Geometry check sheet. Reference: the model listing, model coordinates, mm. Give positions to 0.01 mm unless a question says otherwise; leave off trailing zeros. Order: outer loops, then holes, each group sorted by start corner. A loop starts at its lowest first (then second) coordinate and runs counter-clockwise, first axis right, second up.
Autodesk Inventor part; units mm, degrees
ref_plane "YZ Plane" through (0, 0, 0) normal (1, 0, 0) x (0, 1, 0)
ref_plane "XZ Plane" through (0, 0, 0) normal (0, 1, 0) x (-1, 0, 0)
ref_plane "XY Plane" through (0, 0, 0) normal (0, 0, 1) x (1, 0, 0)
sketch "Sketch1" plane through (0, 0, 0) normal (0, 1, 0) x (-1, 0, 0)
  circle A0 centre (0, 0) radius 2.5
  line L0 (-22.4, 0) -> (15.4, 0)
  line L1 (2.5, 0) -> (1.5, 0)
  line L2 (1.5, 0) -> (1.5, -17)
  line L3 (1.5, -17) -> (2.5, -17)
  line L4 (2.5, -17) -> (2.5, 0)
  line L5 (0, 0) -> (-7.0711, -7.0711) construction
  line L6 (0, 0) -> (10, 0) construction
  line L7 (0, 1.5) -> (-17, 1.5)
  line L8 (-17, 1.5) -> (-17, 2.5)
  line L9 (-17, 2.5) -> (0, 2.5)
  line L10 (0, 1.5) -> (0, 2.5)
  dimension "d0" = 5
  dimension "d1" = 1
  dimension "d2" = 17
  dimension "d3" = 10
  dimension "d4" = 135
extrude "Extrusion1" add sketch "Sketch1" along normal blind 60
sketch "Sketch2" plane through (17, 0, 1.5) normal (0, 0, -1) x (-1, 0, 0)
  line L0 (0, 60) -> (15, 60)
  line L1 (7, 60) -> (7, 0) construction
  line L2 (15, 0) -> (0, 0)
  line L3 (0, 0) -> (0, 60)
  point P0 (17, 0)
  point P1 (7, 30)
  point P2 (7, 53)
  point P3 (7, 7)
  dimension "d7" = 7
  dimension "d8" = 30
  dimension "d9" = 7
  dimension "d10" = 7
hole "Hole1" at (10, 30, 1.5) at (10, 53, 1.5) at (10, 7, 1.5) direction (0, 0, 1) diameter 3.4 end through all
sketch "Sketch3" plane through (-1.5, 0, -2) normal (1, 0, 0) x (0, 0, -1)
  line L0 (0, 60) -> (15, 60)
  line L1 (8, 60) -> (8, 0) construction
  line L2 (15, 0) -> (15, 60)
  line L3 (15, 0) -> (0, 0)
  point P0 (-2, 0)
  point P1 (8, 30)
  point P2 (8, 7)
  point P3 (8, 53)
  dimension "d18" = 7
  dimension "d19" = 30
  dimension "d20" = 7
  dimension "d21" = 7
hole "Hole2" at (-1.5, 30, -10) at (-1.5, 7, -10) at (-1.5, 53, -10) direction (-1, 0, 0) diameter 3.4 end through all
properties part number "scharnier"
Item 1: Sectioned sample at C-C (x = 10). Enter the section's corners in (y, z), and give its area (3 significant figures).
Reported:
outline: (0, 1.5) - (5.3, 1.5) - (5.3, 2.5) - (0, 2.5) - close; (8.7, 1.5) - (28.3, 1.5) - (28.3, 2.5) - (8.7, 2.5) - close; (31.7, 1.5) - (51.3, 1.5) - (51.3, 2.5) - (31.7, 2.5) - close; (54.7, 1.5) - (60, 1.5) - (60, 2.5) - (54.7, 2.5) - close
area: 49.8 mm2
Item 2: Draft check along Z on faces 1 (the cylindrical face through (1.732, 29.58, -1.803)), 2 (the cylindrical face through (11.66, 6.63, 2.01)), 3 (the flat face through (-2, 30, -17)). Enter one of: released by +Z, released by -Z, zero draft, split by the parting line, or undercut.
Reported:
face 1: undercut
face 2: zero draft
face 3: released by -Z
Item 3: Gauge pin test, flat ends, axial feed: pin 1 (4.5 mm diameter, centred on x = 12.5, y = 24, fed in from -Z); pin 2 (4 mm diameter, centred on y = 53, z = -10, fed in from +X); pin 3 (5 mm diameter, centred on x = 2, y = 38, fed in from -Z). Record the tip position at first contact, or that the pin passes through.
Reported:
pin 1: stops at z = 1.5
pin 2: stops at x = -1.5
pin 3: stops at z = -2.5
Item 4: Scan lines: L1, parallel to Y at x = 10, z = 2.3; L2, parallel to X at y = 16.5, z = -12.5; L3, parallel to Z at x = 14.25, y = 12. Record each from-to range of solid material in increasing order.
Reported:
L1: y = 0 to 5.3, 8.7 to 28.3, 31.7 to 51.3, 54.7 to 60
L2: x = -2.5 to -1.5
L3: z = 1.5 to 2.5
Item 5: Sectioned sample at D-D (z = -7.5). Enter the section's corners in (x, y).
Reported:
outline: (-2.5, 0) - (-1.5, 0) - (-1.5, 60) - (-2.5, 60) - close
Item 6: Sectioned sample at B-B (z = -10). Enter the section's corners in (x, y).
Reported:
outline: (-2.5, 0) - (-1.5, 0) - (-1.5, 5.3) - (-2.5, 5.3) - close; (-2.5, 8.7) - (-1.5, 8.7) - (-1.5, 28.3) - (-2.5, 28.3) - close; (-2.5, 31.7) - (-1.5, 31.7) - (-1.5, 51.3) - (-2.5, 51.3) - close; (-2.5, 54.7) - (-1.5, 54.7) - (-1.5, 60) - (-2.5, 60) - close
Item 7: Sectioned sample at A-A (y = 7). Enter the section's corners in (x, z).
Reported:
outline: (-2.5, -17) - (-1.5, -17) - (-1.5, -11.7) - (-2.5, -11.7) - close; (-2.5, -8.3) - (-1.5, -8.3) - (-1.5, -2) arc R2.5 ccw to (2, 1.5) - (8.3, 1.5) - (8.3, 2.5) - (0, 2.5) arc R2.5 ccw to (-2.5, 0) - close; (11.7, 1.5) - (17, 1.5) - (17, 2.5) - (11.7, 2.5) - close
